from build123d import *

# Parameters (mm, degrees)
SKETCH1_W           = 20.86
SKETCH1_H           = 13.2
BOSS_EXTRUDE1_DEPTH = 5.08
SKETCH2_R           = 0.225
BOSS_EXTRUDE2_DEPTH = 6.35
FILLET1_R           = 1


with BuildPart() as part:
    # Sketch1 → Boss-Extrude1 (new body)
    with BuildSketch(Plane.XY):
        with Locations((10.43, 6.6)):
            Rectangle(SKETCH1_W, SKETCH1_H)
    extrude(amount=BOSS_EXTRUDE1_DEPTH)

    # Sketch2 → Boss-Extrude2 (add)
    with BuildSketch(Plane.XY.offset(5.08)):
        with Locations(Location((2.81, 10.41, 0), (0, 0, 180))):
            Circle(SKETCH2_R)
        with Locations(Location((18.05, 10.41, 0), (0, 0, 180))):
            Circle(SKETCH2_R)
        with Locations(Location((18.05, 2.79, 0), (0, 0, 180))):
            Circle(SKETCH2_R)
        with Locations(Location((2.81, 2.79, 0), (0, 0, 180))):
            Circle(SKETCH2_R)
    extrude(amount=BOSS_EXTRUDE2_DEPTH)

    # Fillet1
    fillet1_edges = [part.edges().sort_by_distance(p)[0] for p in [
        (0, 13.2, 2.54),
        (20.86, 0, 2.54),
        (0, 0, 2.54),
    ]]
    fillet(fillet1_edges, radius=FILLET1_R)


solid = part.part
For this review, take the finished solid that the model builds, in its own axes (mm). Round coordinates to 2 decimals unless told otherwise and drop trailing zeros. Write each loop counter-clockwise with the first axis right and the second up, starting at its lowest first coordinate (ties: lowest second). Pieces come first, ordered by that corner, then holes. Notation, with made-up numbers: (-14.5, 85) -> (17.5, 85) arc R30 cw to (17.5, 118) -> close; hole circle Ø7 at (-7.75, 70.25). An arc over 180 degrees is marked (long way). Use CSV: the item, a comma, the result in double quotes.
(1) To check wall thickness, follow L1, parallel to X at y = 12.25, z = 1; L2, parallel to Z at x = 5, y = 3; L3, parallel to X at y = 0.5, z = 3.5. State the ranges of each line that lie inside material, in increasing order. Write a range as [from, to].
Computed values:
L1,"[0, 20.86]"
L2,"[0, 5.08]"
L3,"[0.13, 20.73]"
(2) Consider section A-A, the plane x = 18.05. Give the boundary of the cut face in (y, z) (3 decimals), plus the area to 3 significant figures.
Computed values:
outline,"(0, 0) -> (13.2, 0) -> (13.2, 5.08) -> (10.635, 5.08) -> (10.635, 11.43) -> (10.185, 11.43) -> (10.185, 5.08) -> (3.015, 5.08) -> (3.015, 11.43) -> (2.565, 11.43) -> (2.565, 5.08) -> (0, 5.08) -> close"
area,"72.8 mm²"
(3) Consider section D-D, the plane y = 8. Give the boundary of the cut face in (x, z), plus the area to 3 significant figures.
Computed values:
outline,"(0, 0) -> (20.86, 0) -> (20.86, 5.08) -> (0, 5.08) -> close"
area,"106 mm²"
(4) Consider section C-C, the plane z = 8.5. Give the boundary of the cut face in (x, y) (3 decimals).
Computed values:
outline,"circle Ø0.45 at (2.81, 2.79); circle Ø0.45 at (2.81, 10.41); circle Ø0.45 at (18.05, 2.79); circle Ø0.45 at (18.05, 10.41)"
(5) Clearance check with flat-ended pins moving along their axes: P1, Ø2, axis at x = 10.5, z = 7.5, coming from the -Y side; P2, Ø3, axis at x = 12, y = 8.5, coming from the +Z side; P3, Ø6, axis at y = 11.5, z = 10, coming from the +X side (3 decimals). State where each tip first meets the part, or that it passes through.
Computed values:
P1,"through"
P2,"z = 5.08"
P3,"x = 18.275"
(6) Consider section B-B, the plane y = 2.79. Give the boundary of the cut face in (x, z) (3 decimals), plus the area to 3 significant figures.
Computed values:
outline,"(0, 0) -> (20.86, 0) -> (20.86, 5.08) -> (18.275, 5.08) -> (18.275, 11.43) -> (17.825, 11.43) -> (17.825, 5.08) -> (3.035, 5.08) -> (3.035, 11.43) -> (2.585, 11.43) -> (2.585, 5.08) -> (0, 5.08) -> close"
area,"112 mm²"
